Geometry check sheet. Reference: the model listing, model coordinates, mm. A direction names the side the tool comes from. Give positions to 0.01 mm unless a question says otherwise; leave off trailing zeros. Loops run counter-clockwise (first coordinate to the right, second up) from the corner with the lowest first, then second, coordinate; pieces in that order, holes last. Notation, with made-up numbers: (33.5, 52.25) -> (52.5, 52.25) arc R21 cw to (52.5, 91.25) -> close; hole circle Ø11 at (56.25, 11.25). An arc over 180 degrees is marked (long way). Answer as a JSON object with one key per item and string values.
from build123d import *

# Parameters (mm, degrees)
F0_W           = 1473.2
F0_H           = 279.4
F1_DEPTH       = 12.7
F3_DEPTH       = 279.4
F4_SIZE        = 5.08
F6_D           = 4.826
F6_CBORE_D     = 8.128
F6_CBORE_DEPTH = 4.572


with BuildPart() as f1:
    # F0 (on Front) → F1 (new body)
    with BuildSketch(Plane.XZ):
        Rectangle(F0_W, F0_H)
    extrude(amount=F1_DEPTH)

    # F2 (on face) → F3 (join)
    with BuildSketch(Plane.XY.offset(139.7)):
        Polygon((-731.3394877579, -12.7), (-736.6, -12.7), (-736.6, 0), (-996.9017039253, -260.3017039253), (-969.9609355621, -251.3214478042), align=None)
    extrude(amount=-F3_DEPTH)

    # F4
    f4_edges = [f1.edges().sort_by_distance(p)[0] for p in [
        (-736.6, 0, 0),
        (-731.339488, -12.7, 0),
    ]]
    chamfer(f4_edges, length=F4_SIZE)

    # F6 (through all)
    with Locations(Plane.XZ.offset(12.7)):
        with Locations((279.4, 69.85), (279.4, -69.85), (584.2, -69.85), (584.2, 69.85)):
            CounterBoreHole(F6_D / 2, F6_CBORE_D / 2, F6_CBORE_DEPTH)


solid = f1.part
1) Tool access check on faces 1 (the face through (-5, -12.7, 2)), 2 (the face through (-866.7, -130.1, 2)). Record the directions out of +Z, -Z, +X, -X, +Y, -Y that give a thin tool (end or side, any length) a straight path to the whole face; none if there is none.
Geometry check:
{"face 1": "+Z, -Z, +X, -Y", "face 2": "+Z, -Z, -X, +Y"}
2) Section check A-A on z = 45. Record the cut outline in (x, y), plus the area to 3 significant figures.
Geometry check:
{"outline": "(-996.9, -260.3) -> (-969.96, -251.32) -> (-734.93, -16.29) -> (-726.26, -12.7) -> (736.6, -12.7) -> (736.6, 0) -> (-731.52, 0) -> (-740.19, -3.59) -> close", "area": "23,200 mm2"}
3) Depth check by flat-ended pin: P1, Ø1.5, axis at x = -683.5, z = 58, coming from the -Y side; P2, Ø5, axis at x = -802, z = -8.5, coming from the +Y side; P3, Ø6.5, axis at x = 584.2, z = 69.85, coming from the -Y side. Enter the tip coordinate at first touch or a pass-through.
Geometry check:
{"P1": "stops at y = -12.7", "P2": "stops at y = -62.9", "P3": "stops at y = -8.13"}
4) Material ranges on line 1 along Z through (x, y) = (279, -10); line 2 along Z through (x, y) = (584, -3); line 3 along X through (y, z) = (-11, -69), recorded low to high. Write a range as from..to.
Geometry check:
{"line 1": "z = -139.7..-73.89, -65.81..65.81, 73.89..139.7", "line 2": "z = -139.7..-72.25, -67.45..67.45, 72.25..139.7", "line 3": "x = -747.6..275.43, 283.37..580.23, 588.17..736.6"}
5) Section check B-B on x = 257. Record the cut outline in (y, z), plus the area to 3 significant figures.
Geometry check:
{"outline": "(-12.7, -139.7) -> (0, -139.7) -> (0, 139.7) -> (-12.7, 139.7) -> close", "area": "3,550 mm2"}
6) Section check C-C on y = -106.5. Record the cut outline in (x, z).
Geometry check:
{"outline": "(-843.1, -139.7) -> (-825.14, -139.7) -> (-825.14, 139.7) -> (-843.1, 139.7) -> close"}
